```python
from build123d import *

# Parameters (mm, degrees)
F0_R     = 4.25
F0_R_2   = 5.25
F1_DEPTH = 20


with BuildPart() as f1:
    # F0 (on Top) → F1 (new body)
    with BuildSketch(Plane.XY):
        with BuildLine():
            Line((-193.823792, 58.811097), (-203.820433, -16.185588))
            ThreePointArc((-203.820433, -16.185588), (-201.933428, -22.43342), (-195.989693, -25.129382))
            Line((-195.989693, -25.129382), (-47.989693, -25.129382))
            ThreePointArc((-47.989693, -25.129382), (-41.860303, -22.213415), (-40.255748, -15.618138))
            Line((-40.255748, -15.618138), (-50.236344, 32.288557))
            ThreePointArc((-50.236344, 32.288557), (-52.328942, 36.281327), (-56.264514, 38.479611))
            Line((-56.264514, 38.479611), (-121.196228, 52.174278))
            Line((-121.196228, 52.174278), (-184.268519, 65.476777))
            ThreePointArc((-184.268519, 65.476777), (-190.512926, 64.246558), (-193.823792, 58.811097))
        make_face()
        with Locations((-195.989693, -17.229382)):
            Circle(F0_R, mode=Mode.SUBTRACT)
        with Locations((-179.991815, 8.77348)):
            Circle(F0_R_2, mode=Mode.SUBTRACT)
        with Locations((-47.989693, -17.229382)):
            Circle(F0_R, mode=Mode.SUBTRACT)
        with Locations((-67.991815, 8.765908)):
            Circle(F0_R_2, mode=Mode.SUBTRACT)
        with Locations((-185.993052, 57.767303)):
            Circle(F0_R, mode=Mode.SUBTRACT)
        with Locations((-57.989047, 30.770137)):
            Circle(F0_R, mode=Mode.SUBTRACT)
    extrude(amount=F1_DEPTH)


solid = f1.part
```
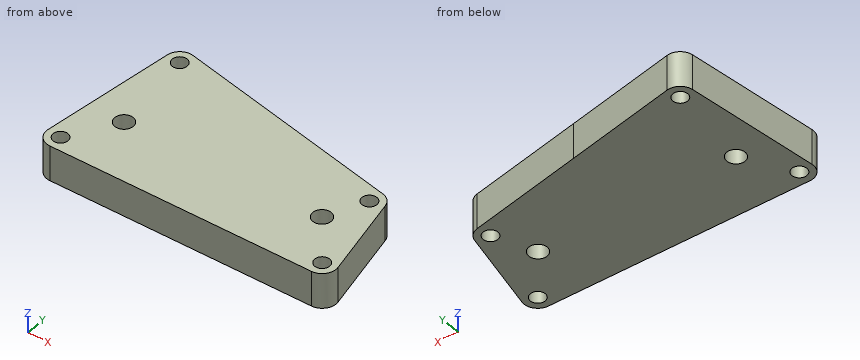
Geometry check sheet. Reference: the model listing, model coordinates, mm. Give positions to 0.01 mm unless a question says otherwise; leave off trailing zeros. Loops run counter-clockwise (first coordinate to the right, second up) from the corner with the lowest first, then second, coordinate; pieces in that order, holes last. Notation, with made-up numbers: M 80.25,70 L 125.25,70 A23 ccw 125.25,101 Z; hole C -25.5,25.25 d9. An arc over 180 degrees is marked long. Write item = value, one per line.
(1) Sectioned sample at B-B, the plane z = 14.75. Record the cut outline in (x, y).
Answer below:
outline = M -203.82,-16.19 A7.9 ccw -195.99,-25.13 L -47.99,-25.13 A7.9 ccw -40.26,-15.62 L -50.24,32.29 A7.9 ccw -56.26,38.48 L -184.27,65.48 A7.9 ccw -193.82,58.81 Z; hole C -195.99,-17.23 d8.5; hole C -185.99,57.77 d8.5; hole C -179.99,8.77 d10.5; hole C -67.99,8.77 d10.5; hole C -57.99,30.77 d8.5; hole C -47.99,-17.23 d8.5
(2) Sectioned sample at C-C, the plane y = 60.5. Record the cut outline in (x, z).
Answer below:
outline = M -193.41,0 L -189.25,0 L -189.25,20 L -193.41,20 Z; M -182.74,0 L -160.67,0 L -160.67,20 L -182.74,20 Z
(3) Material ranges on line 1 (X direction, y = -19, z = 7.75); line 2 (X direction, y = 4.5, z = 18.75); line 3 (X direction, y = 34, z = 13.25), recorded low to high. Write a range as [from, to].
Answer below:
line_1 = [-203.69, -199.85], [-192.13, -51.85], [-44.13, -40.29]
line_2 = [-201.06, -183.04], [-176.94, -71.05], [-64.93, -44.45]
line_3 = [-197.13, -60.75], [-55.23, -50.78]
(4) Gauge pin test, flat ends, axial feed: pin 1 Ø10 at (x, y) = (-195.99, -17.23) entering from -Z; pin 2 Ø8.5 at (x, y) = (-67.99, 8.77) entering from -Z; pin 3 Ø6 at (y, z) = (41.5, 6) entering from -X; pin 4 Ø6 at (y, z) = (14, 15) entering from -X. Record the tip position at first contact, or that the pin passes through.
Answer below:
pin_1 = 0
pin_2 = through
pin_3 = -196.53
pin_4 = -200.2
(5) Sectioned sample at A-A, the plane x = -59. Record the cut outline in (y, z), plus the area to 3 significant figures.
Answer below:
outline = M -25.13,0 L 26.64,0 L 26.64,20 L -25.13,20 Z; M 34.9,0 L 39.06,0 L 39.06,20 L 34.9,20 Z
area = 1,120 mm2
(6) Sectioned sample at D-D, the plane x = -78. Record the cut outline in (y, z).
Answer below:
outline = M -25.13,0 L 43.06,0 L 43.06,20 L -25.13,20 Z
